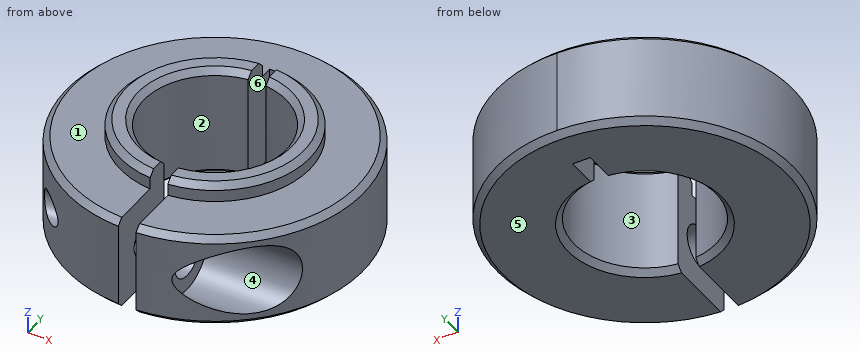
Autodesk Inventor part; units mm, degrees
ref_plane "body_screw_XY" through (3, -9, 0) normal (1, 0, 0) x (0, 0, -1)
ref_plane "body_screw_YZ" through (3, -9, 0) normal (0, 0, -1) x (0, 1, 0)
ref_plane "body_screw_ZX" through (3, -9, 0) normal (0, 1, 0) x (1, 0, 0)
sketch "Sketch_1" plane through (0, 0, 0) normal (1, 0, 0) x (0, 1, 0)
  line L0 (0, -4) -> (0, 5.5)
  line L1 (7.5, 5.5) -> (6.5, 5.5)
  line L2 (6.5, 5.5) -> (6, 5)
  line L3 (6, 5) -> (6, -3.5)
  line L4 (6, -3.5) -> (6.5, -4)
  line L5 (6.5, -4) -> (12, -4)
  line L6 (12, -4) -> (12.5, -3.5)
  line L7 (12.5, -3.5) -> (12.5, 3.5)
  line L8 (12.5, 3.5) -> (12, 4)
  line L9 (12, 4) -> (8, 4)
  line L10 (8, 4) -> (8, 5)
  line L11 (8, 5) -> (7.5, 5.5)
revolve "Revolution1" add sketch "Sketch_1" angle 360 about axis through (0, 0, -4) along (0, 0, -1)
sketch "Sketch_2" plane through (0, 0, 0) normal (0, 0, 1) x (1, 0, 0)
  line L0 (-0.75, -12.5) -> (0.75, -12.5)
  line L1 (0.75, -12.5) -> (0.75, 9)
  line L2 (0.75, 9) -> (-0.75, 9)
  line L3 (-0.75, 9) -> (-0.75, -12.5)
extrude "Extrusion1" cut sketch "Sketch_2" along normal mid plane 32
sketch "Sketch_3" plane through (0, 0, 0) normal (0, 0, 1) x (1, 0, 0)
  line L0 (0, -9) -> (12.5, -9)
  line L1 (12.5, -9) -> (12.5, -12)
  line L2 (12.5, -12) -> (3, -12)
  line L3 (3, -12) -> (3, -10.75)
  line L4 (3, -10.75) -> (0, -10.75)
  line L5 (0, -10.75) -> (0, -9)
  line L6 (0, -9) -> (12.5, -9)
revolve "Revolution2" cut sketch "Sketch_3" angle 360 about axis through (0, -9, 0) along (1, 0, 0)
sketch "Sketch4" plane through (-0.75, -11.9765, -4) normal (1, 0, 0) x (0, 0, -1)
  point P0 (-4, 2.9765)
hole "Hole1" at (-0.75, -9, 0) direction (-1, 0, 0) diameter 2.459 depth 13.5
ref_plane "body_screw_XY" through (3, -9, 0) normal (1, 0, 0) x (0, 0, -1)
ref_plane "body_screw_YZ" through (3, -9, 0) normal (0, 0, -1) x (0, 1, 0)
ref_plane "body_screw_ZX" through (3, -9, 0) normal (0, 1, 0) x (1, 0, 0)
properties part number "SCSNAJ12-16b"
For this review, take the finished solid that the model builds, in its own axes (mm). Face numbers are marked on the shaded views. A direction names the side the tool comes from. Round coordinates to 2 decimals unless told otherwise and drop trailing zeros. Order: outer loops, then holes, each group sorted by start corner. A loop starts at its lowest first (then second) coordinate and runs counter-clockwise, first axis right, second up. Notation, with made-up numbers: (51, -28.5) -> (94, -28.5) arc R9 cw to (94, -24.5) -> close; hole circle Ø9 at (58, 46). An arc over 180 degrees is marked (long way). Write item = value, one per line. Start each with the question number.
1) Insertion check: pin 1 (4 mm diameter, centred on y = -9, z = 0, fed in from +X); pin 2 (2 mm diameter, centred on x = 7, z = 3, fed in from -Y); pin 3 (2 mm diameter, centred on x = 9.5, z = -1.5, fed in from -Y). Each pin has a flat end and moves straight along its axis. Give the tip position at first contact, or say it passes through.
2) Take a section at C-C on x = -4.5. Count the separate pieces of the cut face and the enclosed holes in it, plus the area to 3 significant figures.
3) Take a section at D-D on z = 2.5. State the section outline as (x, y) points.
4) Tool access review of the marked faces 3, 4, 5 and 6: name each direction out of +Z, -Z, +X, -X, +Y, -Y from which nothing blocks a thin tool from reaching the whole face with its end or side.
5) Take a section at A-A on y = 0. State the section outline as (x, z) points.
6) To check wall thickness, follow line 1 (Z direction, x = -4, y = -9); line 2 (Y direction, x = -4.25, z = 0); line 3 (Z direction, x = 7.75, y = -9). State the ranges of each line that lie inside material, in increasing order. Write a range as from..to.
7) Take a section at B-B on z = 0. State the section outline as (x, y) points.
8) The part is to be moulded in two halves that separate along X. For the marked faces 1 and 2, say which applies: +X half, -X half, draft (parallel to the pull), parting line (faces both ways), or undercut.
Verdict:
q1.pin_1 = 3
q1.pin_2 = -10.97
q1.pin_3 = -7.34
q2.separate_pieces = 2
q2.enclosed_holes = 1
q2.area = 125 mm2
q3.outline = (-0.75, -12.48) -> (-0.75, -5.95) arc R6 cw to (-0.75, 5.95) -> (-0.75, 9) -> (0.75, 9) -> (0.75, 5.95) arc R6 cw to (0.75, -5.95) -> (0.75, -12.48) arc R12.5 ccw to (6.53, -10.66) -> (3, -10.66) -> (3, -7.34) -> (10.12, -7.34) arc R12.5 ccw (long way) to start
q4.face_3 = +Z, -Z
q4.face_4 = +X
q4.face_5 = -Z, +X, -X, +Y, -Y
q4.face_6 = +Z, -Z, -Y
q5.outline = (-12.5, -3.5) -> (-12, -4) -> (-6.5, -4) -> (-6, -3.5) -> (-6, 5) -> (-6.5, 5.5) -> (-7.5, 5.5) -> (-8, 5) -> (-8, 4) -> (-12, 4) -> (-12.5, 3.5) -> close; (6, -3.5) -> (6.5, -4) -> (12, -4) -> (12.5, -3.5) -> (12.5, 3.5) -> (12, 4) -> (8, 4) -> (8, 5) -> (7.5, 5.5) -> (6.5, 5.5) -> (6, 5) -> close
q6.line_1 = -4..-1.23, 1.23..4
q6.line_2 = -11.76..-10.23, -7.77..-4.24, 4.24..11.76
q6.line_3 = -4..-3, 3..4
q7.outline = (-9.79, -7.77) -> (-0.75, -7.77) -> (-0.75, -5.95) arc R6 cw to (-0.75, 5.95) -> (-0.75, 9) -> (0.75, 9) -> (0.75, 5.95) arc R6 cw to (0.75, -5.95) -> (0.75, -7.25) -> (3, -7.25) -> (3, -6) -> (10.97, -6) arc R12.5 ccw (long way) to start; (-7.18, -10.23) arc R12.5 ccw to (-0.75, -12.48) -> (-0.75, -10.23) -> close; (0.75, -12.48) arc R12.5 ccw to (3.5, -12) -> (3, -12) -> (3, -10.75) -> (0.75, -10.75) -> close
q8.face_1 = draft
q8.face_2 = undercut
